Here's how the part is built. I have some questions about the finished solid (model axes, mm). A direction names the side the tool comes from. Round coordinates to 2 decimals unless told otherwise and drop trailing zeros. Write each loop counter-clockwise with the first axis right and the second up, starting at its lowest first coordinate (ties: lowest second). Pieces come first, ordered by that corner, then holes. Notation, with made-up numbers: (-2, -15.5) -> (2, -15.5) arc R19 ccw to (2, 8.5) -> close; hole circle Ø9 at (36, 18). An arc over 180 degrees is marked (long way). Put each result on its own line as item: value. Start each with the question number.
1) Which directions (+Z, -Z, +X, -X, +Y, -Y) give clear straight access to the entire face, cutting with the end or side of a thin tool? Please do faces 1 (the cylindrical face through (3.974, 13.266, -0.173)), 2 (the flat face through (2, -8, -11.075)), 3 (the cylindrical face through (0.376, 13.266, 0.173)).
2) We'd pull the mould along Y, two halves only. Please class faces 4 (the cylindrical face through (2.16, -17.86, 16.05)), 5 (the cylindrical face through (0.38, -10.56, -16.05)), 6 (the cylindrical face through (0.38, -8.98, -11.43)): released by +Y, released by -Y, zero draft, split by the parting line, or undercut.
3) I want a section at A-A, the plane y = -12. List the corners of the cut face in (x, z) for me (3 decimals), then the cut area to 3 significant figures.
4) If I drill on line 1 along Y through (x, z) = (1.2, -2); line 2 along Z through (x, y) = (1.5, -11) (3 decimals); line 3 along Y through (x, z) = (0.55, -3.5), over which ranges is the centre line in solid material (lowest first)? Write a range as [from, to].
5) I want a section at B-B, the plane z = -8. List the corners of the cut face in (x, y) for me, then the cut area to 3 significant figures.
6) I want a section at D-D, the plane x = 2.55. List the corners of the cut face in (y, z) for me (3 decimals).
7) I want a section at C-C, the plane y = -0.5. List the corners of the cut face in (x, z) for me (3 decimals).
8) Will these pins go through, and if not, where does the flat tip stop? P1, Ø1.5, axis at x = 1, z = 8.5, coming from the -Y side; P2, Ø1.5, axis at y = 7, z = 9.5, coming from the +X side.
from build123d import *

# Parameters (mm, degrees)
BOSS_EXTRUDE1_DEPTH = 4.35
FILLET1_R           = 1.25
FILLET2_R           = 1.25


with BuildPart() as part:
    # Sketch1 → Boss-Extrude1 (new body)
    with BuildSketch(Plane(origin=(0, 0, 0), x_dir=(0, 0, -1), z_dir=(1, 0, 0))):
        with BuildLine():
            Line((-11.075, 12.91), (11.075, 12.91))
            Line((11.075, 12.91), (11.075, 3.951551724))
            ThreePointArc((11.075, 3.951551724), (13.74, 5.077445529), (16.405, 3.951551724))
            Line((16.405, 3.951551724), (16.405, 18.24))
            Line((16.405, 18.24), (-16.405, 18.24))
            Line((-16.405, 18.24), (-16.405, -18.24))
            Line((-16.405, -18.24), (16.405, -18.24))
            Line((16.405, -18.24), (16.405, -3.951551724))
            ThreePointArc((16.405, -3.951551724), (13.74, -5.077445529), (11.075, -3.951551724))
            Line((11.075, -3.951551724), (11.075, -12.91))
            Line((11.075, -12.91), (-11.075, -12.91))
            Line((-11.075, -12.91), (-11.075, 12.91))
        make_face()
    extrude(amount=BOSS_EXTRUDE1_DEPTH)

    # Fillet1
    fillet1_edges = [part.edges().sort_by_distance(p)[0] for p in [
        (4.35, 8.430775862, -11.075),
        (4.35, 11.095775862, -16.405),
        (4.35, 18.24, 0),
        (4.35, 0, 16.405),
        (4.35, -18.24, 0),
        (4.35, -11.095775862, -16.405),
        (4.35, -8.430775862, -11.075),
        (4.35, -12.91, 0),
        (4.35, 0, 11.075),
        (4.35, 12.91, 0),
    ]]
    fillet(fillet1_edges, radius=FILLET1_R)

    # Fillet2
    # the kernel refuses this fillet: 1.25 mm, written as the material it takes off along each edge
    with BuildSketch(Plane(origin=(3.1, -16.99, -15.155), x_dir=(0, -1, 0), z_dir=(0, 0, -1))) as fillet2_piece_1_section:
        Polygon((0, 0), (FILLET2_R, 0), (FILLET2_R, -FILLET2_R), (0, -FILLET2_R), align=None)
    fillet2_piece_1 = extrude(amount=FILLET2_R, mode=Mode.PRIVATE)
    fillet2_piece_1 = fillet2_piece_1 - Plane(origin=(3.1, -16.99, -15.155), x_dir=(-0.7071067811865475, 0.7071067811865475, 0), z_dir=(0, 0, -1)) * Sphere(FILLET2_R, mode=Mode.PRIVATE)
    add(fillet2_piece_1, mode=Mode.SUBTRACT)
    with BuildSketch(Plane(origin=(3.1, -16.99, 15.155), x_dir=(0, -1, 0), z_dir=(0, 0, 1))) as fillet2_piece_2_section:
        Polygon((0, 0), (FILLET2_R, 0), (FILLET2_R, FILLET2_R), (0, FILLET2_R), align=None)
    fillet2_piece_2 = extrude(amount=FILLET2_R, mode=Mode.PRIVATE)
    fillet2_piece_2 = fillet2_piece_2 - Plane(origin=(3.1, -16.99, 15.155), x_dir=(-0.7071067811865475, 0.7071067811865475, 0), z_dir=(0, 0, 1)) * Sphere(FILLET2_R, mode=Mode.PRIVATE)
    add(fillet2_piece_2, mode=Mode.SUBTRACT)
    with BuildSketch(Plane(origin=(1.25, -16.99, -15.155), x_dir=(-1, 0, 0), z_dir=(0, -1, 0))) as fillet2_piece_3_section:
        Polygon((0, 0), (FILLET2_R, 0), (FILLET2_R, FILLET2_R), (0, FILLET2_R), align=None)
    fillet2_piece_3 = extrude(amount=FILLET2_R, mode=Mode.PRIVATE)
    fillet2_piece_3 = fillet2_piece_3 - Plane(origin=(1.25, -16.99, -15.155), x_dir=(0.7071067811865475, 0, 0.7071067811865475), z_dir=(0, -1, 0)) * Sphere(FILLET2_R, mode=Mode.PRIVATE)
    add(fillet2_piece_3, mode=Mode.SUBTRACT)
    with BuildSketch(Plane(origin=(1.25, -16.99, 15.155), x_dir=(-1, 0, 0), z_dir=(0, -1, 0))) as fillet2_piece_4_section:
        Polygon((0, 0), (FILLET2_R, 0), (FILLET2_R, -FILLET2_R), (0, -FILLET2_R), align=None)
    fillet2_piece_4 = extrude(amount=FILLET2_R, mode=Mode.PRIVATE)
    fillet2_piece_4 = fillet2_piece_4 - Plane(origin=(1.25, -16.99, 15.155), x_dir=(0.7071067811865475, 0, -0.7071067811865475), z_dir=(0, -1, 0)) * Sphere(FILLET2_R, mode=Mode.PRIVATE)
    add(fillet2_piece_4, mode=Mode.SUBTRACT)
    with BuildSketch(Plane(origin=(0, -12.91, -11.075), x_dir=(0, -1, 0), z_dir=(0, 0, 1)), Plane(origin=(0, 12.91, 11.075), x_dir=(0, 1, 0), z_dir=(0, 0, -1))) as fillet2_piece_5:
        with BuildLine():
            CenterArc((FILLET2_R, FILLET2_R), FILLET2_R, 180, 90)
            Line((0, FILLET2_R), (0, 0))
            Line((0, 0), (FILLET2_R, 0))
        make_face()
    extrude(amount=22.15, mode=Mode.SUBTRACT)
    with BuildSketch(Plane(origin=(0, -0.826551724, -11.075), x_dir=(1, 0, 0), z_dir=(0, -1, 0))) as fillet2_piece_6:
        with BuildLine():
            CenterArc((FILLET2_R, -FILLET2_R), FILLET2_R, 90, 90)
            Line((0, -FILLET2_R), (0, 0))
            Line((0, 0), (FILLET2_R, 0))
        make_face()
    extrude(amount=12.083448276, mode=Mode.SUBTRACT)
    with BuildSketch(Plane(origin=(0, -16.99, -16.405), x_dir=(0, 0, 1), z_dir=(0, 1, 0))) as fillet2_piece_7:
        with BuildLine():
            CenterArc((FILLET2_R, FILLET2_R), FILLET2_R, 180, 90)
            Line((0, FILLET2_R), (0, 0))
            Line((0, 0), (FILLET2_R, 0))
        make_face()
    extrude(amount=16.163448276, mode=Mode.SUBTRACT)
    with BuildSketch(Plane(origin=(0, -18.24, 15.155), x_dir=(0, 1, 0), z_dir=(0, 0, -1))) as fillet2_piece_8:
        with BuildLine():
            CenterArc((FILLET2_R, FILLET2_R), FILLET2_R, 180, 90)
            Line((0, FILLET2_R), (0, 0))
            Line((0, 0), (FILLET2_R, 0))
        make_face()
    extrude(amount=30.31, mode=Mode.SUBTRACT)
    with BuildSketch(Plane(origin=(0, 21.365, 16.405), x_dir=(0, 0, -1), z_dir=(0, -1, 0))) as fillet2_piece_9:
        with BuildLine():
            CenterArc((FILLET2_R, FILLET2_R), FILLET2_R, 180, 90)
            Line((0, FILLET2_R), (0, 0))
            Line((0, 0), (FILLET2_R, 0))
        make_face()
    extrude(amount=38.355, mode=Mode.SUBTRACT)
    with BuildSketch(Plane(origin=(0, 18.24, -19.53), x_dir=(0, -1, 0), z_dir=(0, 0, 1))) as fillet2_piece_10:
        with BuildLine():
            CenterArc((FILLET2_R, FILLET2_R), FILLET2_R, 180, 90)
            Line((0, FILLET2_R), (0, 0))
            Line((0, 0), (FILLET2_R, 0))
        make_face()
    extrude(amount=39.06, mode=Mode.SUBTRACT)
    with BuildSketch(Plane(origin=(0, 0.826551724, -16.405), x_dir=(0, 0, 1), z_dir=(0, 1, 0))) as fillet2_piece_11:
        with BuildLine():
            CenterArc((FILLET2_R, FILLET2_R), FILLET2_R, 180, 90)
            Line((0, FILLET2_R), (0, 0))
            Line((0, 0), (FILLET2_R, 0))
        make_face()
    extrude(amount=20.538448276, mode=Mode.SUBTRACT)
    with BuildSketch(Plane(origin=(0, 12.91, -11.075), x_dir=(0, 0, -1), z_dir=(0, -1, 0))) as fillet2_piece_12:
        with BuildLine():
            CenterArc((FILLET2_R, FILLET2_R), FILLET2_R, 180, 90)
            Line((0, FILLET2_R), (0, 0))
            Line((0, 0), (FILLET2_R, 0))
        make_face()
    extrude(amount=12.083448276, mode=Mode.SUBTRACT)
    with BuildSketch(Plane(origin=(0, -12.91, 11.075), x_dir=(0, 0, 1), z_dir=(0, 1, 0))) as fillet2_piece_13:
        with BuildLine():
            CenterArc((FILLET2_R, FILLET2_R), FILLET2_R, 180, 90)
            Line((0, FILLET2_R), (0, 0))
            Line((0, 0), (FILLET2_R, 0))
        make_face()
    extrude(amount=25.82, mode=Mode.SUBTRACT)
    with BuildSketch(Plane(origin=(1.25, -18.24, 16.405), x_dir=(0, 1, 0), z_dir=(1, 0, 0))) as fillet2_piece_14:
        with BuildLine():
            CenterArc((FILLET2_R, -FILLET2_R), FILLET2_R, 90, 90)
            Line((0, -FILLET2_R), (0, 0))
            Line((0, 0), (FILLET2_R, 0))
        make_face()
    extrude(amount=1.85, mode=Mode.SUBTRACT)
    with BuildSketch(Plane(origin=(1.25, -18.24, -16.405), x_dir=(0, 1, 0), z_dir=(1, 0, 0))) as fillet2_piece_15:
        with BuildLine():
            CenterArc((FILLET2_R, FILLET2_R), FILLET2_R, 180, 90)
            Line((0, FILLET2_R), (0, 0))
            Line((0, 0), (FILLET2_R, 0))
        make_face()
    extrude(amount=1.85, mode=Mode.SUBTRACT)
    with BuildSketch(Plane(origin=(0, -0.826551724, -11.075), x_dir=(1, 0, 0), z_dir=(0, -1, 0))) as fillet2_piece_16a_section:
        with BuildLine():
            CenterArc((FILLET2_R, -FILLET2_R), FILLET2_R, 90, 90)
            Line((0, -FILLET2_R), (0, 0))
            Line((0, 0), (FILLET2_R, 0))
        make_face()
    fillet2_piece_16a = extrude(amount=15.208448276, mode=Mode.PRIVATE)
    fillet2_piece_16a = split(fillet2_piece_16a, bisect_by=Plane(origin=(0.282993893, -12.91, -11.357993893), z_dir=(0, -1, 0)), keep=Keep.TOP, mode=Mode.PRIVATE)
    with BuildSketch(Plane(origin=(0, -12.91, -14.2), x_dir=(0, -1, 0), z_dir=(0, 0, 1))) as fillet2_piece_16b_section:
        with BuildLine():
            CenterArc((FILLET2_R, FILLET2_R), FILLET2_R, 180, 90)
            Line((0, FILLET2_R), (0, 0))
            Line((0, 0), (FILLET2_R, 0))
        make_face()
    fillet2_piece_16b = extrude(amount=25.275, mode=Mode.PRIVATE)
    fillet2_piece_16b = split(fillet2_piece_16b, bisect_by=Plane(origin=(0.282993893, -13.192993893, -11.075), z_dir=(0, 0, -1)), keep=Keep.TOP, mode=Mode.PRIVATE)
    fillet2_piece_16 = fillet2_piece_16a & fillet2_piece_16b
    add(fillet2_piece_16, mode=Mode.SUBTRACT)
    with BuildSketch(Plane(origin=(0, -12.91, -11.075), x_dir=(0, -1, 0), z_dir=(0, 0, 1))) as fillet2_piece_17a_section:
        with BuildLine():
            CenterArc((FILLET2_R, FILLET2_R), FILLET2_R, 180, 90)
            Line((0, FILLET2_R), (0, 0))
            Line((0, 0), (FILLET2_R, 0))
        make_face()
    fillet2_piece_17a = extrude(amount=25.275, mode=Mode.PRIVATE)
    fillet2_piece_17a = split(fillet2_piece_17a, bisect_by=Plane(origin=(0.282993893, -13.192993893, 11.075), z_dir=(0, 0, 1)), keep=Keep.TOP, mode=Mode.PRIVATE)
    with BuildSketch(Plane(origin=(0, -16.035, 11.075), x_dir=(0, 0, 1), z_dir=(0, 1, 0))) as fillet2_piece_17b_section:
        with BuildLine():
            CenterArc((FILLET2_R, FILLET2_R), FILLET2_R, 180, 90)
            Line((0, FILLET2_R), (0, 0))
            Line((0, 0), (FILLET2_R, 0))
        make_face()
    fillet2_piece_17b = extrude(amount=28.945, mode=Mode.PRIVATE)
    fillet2_piece_17b = split(fillet2_piece_17b, bisect_by=Plane(origin=(0.282993893, -12.91, 11.357993893), z_dir=(0, -1, 0)), keep=Keep.TOP, mode=Mode.PRIVATE)
    fillet2_piece_17 = fillet2_piece_17a & fillet2_piece_17b
    add(fillet2_piece_17, mode=Mode.SUBTRACT)
    with BuildSketch(Plane(origin=(0, 12.91, 11.075), x_dir=(0, 1, 0), z_dir=(0, 0, -1))) as fillet2_piece_18a_section:
        with BuildLine():
            CenterArc((FILLET2_R, FILLET2_R), FILLET2_R, 180, 90)
            Line((0, FILLET2_R), (0, 0))
            Line((0, 0), (FILLET2_R, 0))
        make_face()
    fillet2_piece_18a = extrude(amount=25.275, mode=Mode.PRIVATE)
    fillet2_piece_18a = split(fillet2_piece_18a, bisect_by=Plane(origin=(0.282993893, 13.192993893, -11.075), z_dir=(0, 0, -1)), keep=Keep.TOP, mode=Mode.PRIVATE)
    with BuildSketch(Plane(origin=(0, 16.035, -11.075), x_dir=(0, 0, -1), z_dir=(0, -1, 0))) as fillet2_piece_18b_section:
        with BuildLine():
            CenterArc((FILLET2_R, FILLET2_R), FILLET2_R, 180, 90)
            Line((0, FILLET2_R), (0, 0))
            Line((0, 0), (FILLET2_R, 0))
        make_face()
    fillet2_piece_18b = extrude(amount=15.208448276, mode=Mode.PRIVATE)
    fillet2_piece_18b = split(fillet2_piece_18b, bisect_by=Plane(origin=(0.282993893, 12.91, -11.357993893), z_dir=(0, 1, 0)), keep=Keep.TOP, mode=Mode.PRIVATE)
    fillet2_piece_18 = fillet2_piece_18a & fillet2_piece_18b
    add(fillet2_piece_18, mode=Mode.SUBTRACT)
    with BuildSketch(Plane(origin=(0, -12.91, 11.075), x_dir=(0, 0, 1), z_dir=(0, 1, 0))) as fillet2_piece_19a_section:
        with BuildLine():
            CenterArc((FILLET2_R, FILLET2_R), FILLET2_R, 180, 90)
            Line((0, FILLET2_R), (0, 0))
            Line((0, 0), (FILLET2_R, 0))
        make_face()
    fillet2_piece_19a = extrude(amount=28.945, mode=Mode.PRIVATE)
    fillet2_piece_19a = split(fillet2_piece_19a, bisect_by=Plane(origin=(0.282993893, 12.91, 11.357993893), z_dir=(0, 1, 0)), keep=Keep.TOP, mode=Mode.PRIVATE)
    with BuildSketch(Plane(origin=(0, 12.91, 14.2), x_dir=(0, 1, 0), z_dir=(0, 0, -1))) as fillet2_piece_19b_section:
        with BuildLine():
            CenterArc((FILLET2_R, FILLET2_R), FILLET2_R, 180, 90)
            Line((0, FILLET2_R), (0, 0))
            Line((0, 0), (FILLET2_R, 0))
        make_face()
    fillet2_piece_19b = extrude(amount=25.275, mode=Mode.PRIVATE)
    fillet2_piece_19b = split(fillet2_piece_19b, bisect_by=Plane(origin=(0.282993893, 13.192993893, 11.075), z_dir=(0, 0, 1)), keep=Keep.TOP, mode=Mode.PRIVATE)
    fillet2_piece_19 = fillet2_piece_19a & fillet2_piece_19b
    add(fillet2_piece_19, mode=Mode.SUBTRACT)


solid = part.part
Findings:
1. face 1: +X
1. face 2: +X, -X
1. face 3: -X
2. face 4: released by -Y
2. face 5: zero draft
2. face 6: undercut
3. outline: (0, -15.155) arc R1.25 ccw to (1.25, -16.405) -> (3.1, -16.405) arc R1.25 ccw to (4.35, -15.155) -> (4.35, -12.325) arc R1.25 ccw to (3.1, -11.075) -> (1.25, -11.075) arc R1.25 ccw to (0, -12.325) -> close; (0, 12.325) arc R1.25 ccw to (1.25, 11.075) -> (3.1, 11.075) arc R1.25 ccw to (4.35, 12.325) -> (4.35, 15.155) arc R1.25 ccw to (3.1, 16.405) -> (1.25, 16.405) arc R1.25 ccw to (0, 15.155) -> close
3. area: 43.7 mm2
4. line 1: y = [-18.24, -12.91], [12.91, 18.24]
4. line 2: z = [-16.405, -11.075], [11.075, 16.405]
4. line 3: y = [-18.03, -13.12], [13.12, 18.03]
5. outline: (0, -16.99) arc R1.25 ccw to (1.25, -18.24) -> (3.1, -18.24) arc R1.25 ccw to (4.35, -16.99) -> (4.35, -14.16) arc R1.25 ccw to (3.1, -12.91) -> (1.25, -12.91) arc R1.25 ccw to (0, -14.16) -> close; (0, 14.16) arc R1.25 ccw to (1.25, 12.91) -> (3.1, 12.91) arc R1.25 ccw to (4.35, 14.16) -> (4.35, 16.99) arc R1.25 ccw to (3.1, 18.24) -> (1.25, 18.24) arc R1.25 ccw to (0, 16.99) -> close
5. area: 43.7 mm2
6. outline: (-18.24, -15.155) arc R1.25 ccw to (-16.99, -16.405) -> (-3.952, -16.405) arc R3.717 cw to (-3.952, -11.075) -> (-12.91, -11.075) -> (-12.91, 11.075) -> (12.91, 11.075) -> (12.91, -11.075) -> (3.952, -11.075) arc R3.717 cw to (3.952, -16.405) -> (18.24, -16.405) -> (18.24, 16.405) -> (-16.99, 16.405) arc R1.25 ccw to (-18.24, 15.155) -> close
7. outline: (0, 12.325) arc R1.25 ccw to (1.25, 11.075) -> (3.1, 11.075) arc R1.25 ccw to (4.35, 12.325) -> (4.35, 15.155) arc R1.25 ccw to (3.1, 16.405) -> (1.25, 16.405) arc R1.25 ccw to (0, 15.155) -> close
8. P1: stops at y = -18.24
8. P2: passes through
